Input: dimensioned drawing with shaded views. Units: mm. Origin: part minimum x, y, z. A direction names the side the tool comes from. Give positions to 0.01 mm unless a question says otherwise; leave off trailing zeros. Loops run counter-clockwise (first coordinate to the right, second up) from the corner with the lowest first, then second, coordinate; pieces in that order, holes last. Notation, with made-up numbers: M 53,61.5 L 95,61.5 A24 ccw 95,81.5 Z; hole C -28,27.5 d11. An arc over 180 degrees is marked long. Answer in a Markdown table with one row per item.
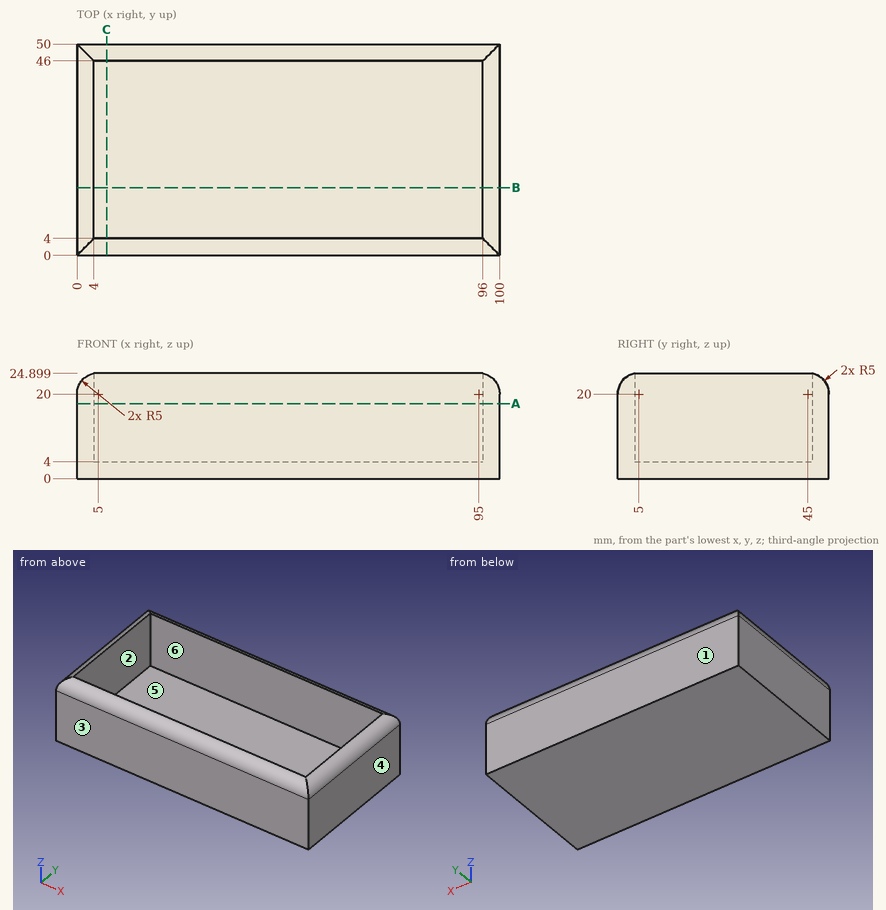
Q1. Mould query, pull axis Y, two halves, no side actions, for the marked faces 3, 4, 5 and 6. Classes: +Y half, -Y half, draft (parallel to the pull), parting line (faces both ways), or undercut.
Values follow:
| item | result |
|---|---|
| face 3 | -Y half |
| face 4 | draft |
| face 5 | undercut |
| face 6 | undercut |
Q2. Section query C-C (x = 7). Output: boundary loops of the cut face in (y, z).
Values follow:
| item | result |
|---|---|
| outline | M 0,0 L 50,0 L 50,20 A5 ccw 46,24.9 L 46,4 L 4,4 L 4,24.9 A5 ccw 0,20 Z |
Q3. Ray query, probe 1 along Y at (x, z) = (70.5, 17); probe 2 along X at (y, z) = (13.5, 13); probe 3 along Z at (x, y) = (72, 45). Return the intervals inside material, ascending. Write a range as from..to.
Values follow:
| item | result |
|---|---|
| probe 1 | 0..4, 46..50 |
| probe 2 | 0..4, 96..100 |
| probe 3 | 0..4 |
Q4. Contact query for flat-ended pins moving along their axis: pin 1 Ø5 at (x, y) = (31, 11.5) entering from -Z; pin 2 Ø10 at (x, y) = (82.5, 8) entering from +Z; pin 3 Ø10 at (x, y) = (83.5, 18.5) entering from +Z. Output: stop coordinate, or through.
Values follow:
| item | result |
|---|---|
| pin 1 | z = 0 |
| pin 2 | z = 24.9 |
| pin 3 | z = 4 |
Q5. Section query A-A (z = 17.75). Output: boundary loops of the cut face in (x, y).
Values follow:
| item | result |
|---|---|
| outline | M 0,0 L 100,0 L 100,50 L 0,50 Z; hole M 4,4 L 96,4 L 96,46 L 4,46 Z |
Q6. Section query B-B (y = 16). Output: boundary loops of the cut face in (x, z), plus the area to 3 significant figures.
Values follow:
| item | result |
|---|---|
| outline | M 0,0 L 100,0 L 100,20 A5 ccw 96,24.9 L 96,4 L 4,4 L 4,24.9 A5 ccw 0,20 Z |
| area | 557 mm^2 |
Q7. Reachability of the marked faces 1 and 2 from +Z, -Z, +X, -X, +Y, -Y: full face, straight path, thin tool, end or side. Return the list, or none.
Values follow:
| item | result |
|---|---|
| face 1 | +Z, -Z, +X, -X, +Y |
| face 2 | +Z |
